from build123d import *

# Parameters (mm, degrees)
SKETCH2_R           = 1.5
CUT_EXTRUDE1_DEPTH  = 10
CUT_EXTRUDE2_DEPTH  = 7
SKETCH4_R           = 2.125
CUT_EXTRUDE4_DEPTH  = 3.5
BOSS_EXTRUDE1_START = 3.7
SKETCH5_R           = 2.1
SKETCH5_R_2         = 1.5
BOSS_EXTRUDE1_DEPTH = 3.7


with BuildPart() as part:
    # Sketch1 → Revolve1 (revolve)
    with BuildSketch(Plane.XY):
        with BuildLine():
            Line((0, 0), (-25, 0))
            ThreePointArc((-25, 0), (-12.85331964, 4.2665982), (0, 5))
            Line((0, 5), (0, 0))
        make_face()
    revolve(axis=Axis((0, 0, 0), (0, 1, 0)))

    # Sketch2 → Cut-Extrude1 (cut)
    with BuildSketch(Plane(origin=(0, 0, 0), x_dir=(-1, 0, 0), z_dir=(0, -1, 0))):
        with Locations(Location((15.4, -10.4, 0), (0, 0, 90))):
            Circle(SKETCH2_R)
        with Locations(Location((-15.4, -10.4, 0), (0, 0, 304.757660669))):
            Circle(SKETCH2_R)
        with Locations(Location((-15.4, 10.4, 0), (0, 0, 90))):
            Circle(SKETCH2_R)
        with Locations(Location((15.4, 10.4, 0), (0, 0, 33.710682562))):
            Circle(SKETCH2_R)
    extrude(amount=-CUT_EXTRUDE1_DEPTH, mode=Mode.SUBTRACT)

    # Sketch3 → Cut-Extrude2 (cut)
    with BuildSketch(Plane(origin=(0, 0, 0), x_dir=(-1, 0, 0), z_dir=(0, -1, 0))):
        with BuildLine():
            Line((11.75, -12.75), (-11.75, -12.75))
            ThreePointArc((-11.75, -12.75), (-12.457106781, -12.457106781), (-12.75, -11.75))
            Line((-12.75, -11.75), (-12.75, 11.75))
            ThreePointArc((-12.75, 11.75), (-12.457106781, 12.457106781), (-11.75, 12.75))
            Line((-11.75, 12.75), (11.75, 12.75))
            ThreePointArc((11.75, 12.75), (12.457106781, 12.457106781), (12.75, 11.75))
            Line((12.75, 11.75), (12.75, -11.75))
            ThreePointArc((12.75, -11.75), (12.457106781, -12.457106781), (11.75, -12.75))
        make_face()
    extrude(amount=-CUT_EXTRUDE2_DEPTH, mode=Mode.SUBTRACT)

    # Sketch4 → Cut-Extrude4 (cut)
    with BuildSketch(Plane(origin=(0, 5, 0), x_dir=(1, 0, 0), z_dir=(0, 1, 0))):
        with Locations(Location((-15.4, 10.4, 0), (0, 0, 270))):
            Circle(SKETCH4_R)
        with Locations(Location((15.4, 10.4, 0), (0, 0, 127.696473345))):
            Circle(SKETCH4_R)
        with Locations(Location((15.4, -10.4, 0), (0, 0, 270))):
            Circle(SKETCH4_R)
        with Locations(Location((-15.4, -10.4, 0), (0, 0, 140.12364515))):
            Circle(SKETCH4_R)
    extrude(amount=-CUT_EXTRUDE4_DEPTH, mode=Mode.SUBTRACT)

    # Sketch5 → Boss-Extrude1 (add)
    # profile 1 of 4: a face of its own
    with BuildSketch(Plane(origin=(0, 0, 0), x_dir=(-1, 0, 0), z_dir=(0, -1, 0)).offset(BOSS_EXTRUDE1_START)):
        with Locations(Location((-15.4, -10.4, 0), (0, 0, 270))):
            Circle(SKETCH5_R)
        with Locations(Location((-15.4, -10.4, 0), (0, 0, 90))):
            Circle(SKETCH5_R_2, mode=Mode.SUBTRACT)
    # profile 2 of 4: a face of its own
    with BuildSketch(Plane(origin=(0, 0, 0), x_dir=(-1, 0, 0), z_dir=(0, -1, 0)).offset(BOSS_EXTRUDE1_START)):
        with Locations(Location((15.4, -10.4, 0), (0, 0, 270))):
            Circle(SKETCH5_R)
        with Locations(Location((15.4, -10.4, 0), (0, 0, 90))):
            Circle(SKETCH5_R_2, mode=Mode.SUBTRACT)
    # profile 3 of 4: a face of its own
    with BuildSketch(Plane(origin=(0, 0, 0), x_dir=(-1, 0, 0), z_dir=(0, -1, 0)).offset(BOSS_EXTRUDE1_START)):
        with Locations(Location((-15.4, 10.4, 0), (0, 0, 270))):
            Circle(SKETCH5_R)
        with Locations(Location((-15.4, 10.4, 0), (0, 0, 90))):
            Circle(SKETCH5_R_2, mode=Mode.SUBTRACT)
    # profile 4 of 4: a face of its own
    with BuildSketch(Plane(origin=(0, 0, 0), x_dir=(-1, 0, 0), z_dir=(0, -1, 0)).offset(BOSS_EXTRUDE1_START)):
        with Locations(Location((15.4, 10.4, 0), (0, 0, 270))):
            Circle(SKETCH5_R)
        with Locations(Location((15.4, 10.4, 0), (0, 0, 90))):
            Circle(SKETCH5_R_2, mode=Mode.SUBTRACT)
    extrude(amount=-BOSS_EXTRUDE1_DEPTH)


solid = part.part
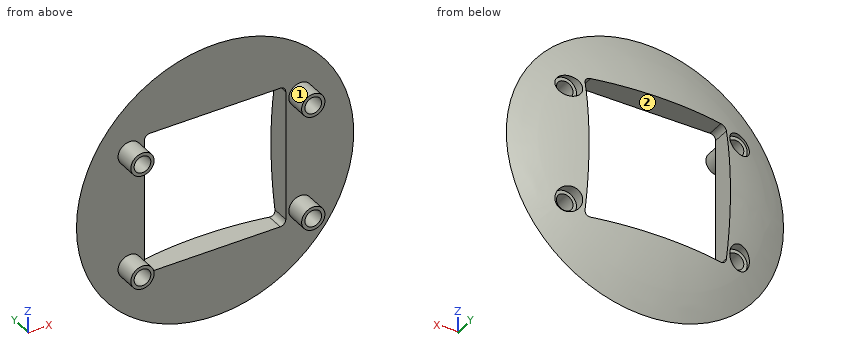
The listing builds one solid part. Answer for the finished solid, in the listing's coordinates (mm). Face numbers are marked on the shaded views. A direction names the side the tool comes from. Give positions to 0.01 mm unless a question says otherwise; leave off trailing zeros. Write each loop counter-clockwise with the first axis right and the second up, starting at its lowest first coordinate (ties: lowest second). Pieces come first, ordered by that corner, then holes. Notation, with made-up numbers: (26, -4.5) -> (34, -4.5) arc R25 ccw to (34, 16.5) -> close; hole circle Ø7 at (-23, 80). An arc over 180 degrees is marked (long way). One line per question, with ' | ' between items. Start each with the question number.
1. Section A-A (y = -2.5) is taken. Determine the outline of the cut face in (x, z), plus the area to 3 significant figures.
2. For the marked faces 1 and 2, determine the directions among +Z, -Z, +X, -X, +Y, -Y from which every point of the face is accessible in a straight line to the end or side of a thin tool.
3. Find the intervals of material crossed by probe 1 along X at (y, z) = (-0.7, 10.4); probe 2 along Z at (x, y) = (-14.5, -0.25); probe 3 along X at (y, z) = (2.3, 10.4) (3 decimals), in increasing order.
4. Given pin 1 Ø4.5 at (x, z) = (-15, 10.5) entering from +Y; pin 2 Ø2 at (y, z) = (2.5, 3) entering from -X; pin 3 Ø2.5 at (x, z) = (15.4, -10.4) entering from +Y; pin 4 Ø15 at (x, z) = (9.5, -0.5) entering from -Y, each flat-ended and moving along its own axis, determine where each tip first touches the part or whether it passes through.
Response values:
1) outline: circle Ø4.2 at (-15.4, -10.4); circle Ø4.2 at (-15.4, 10.4); circle Ø4.2 at (15.4, -10.4); circle Ø4.2 at (15.4, 10.4); hole circle Ø3 at (-15.4, -10.4); hole circle Ø3 at (-15.4, 10.4); hole circle Ø3 at (15.4, -10.4); hole circle Ø3 at (15.4, 10.4) | area: 27.1 mm2
2) face 1: -Y | face 2: +Y, -Y
3) probe 1: -17.5 to -16.9, -13.9 to -13.3, 13.3 to 13.9, 16.9 to 17.5 | probe 2: -12.3 to -11.6, -9.2 to -8.5, 8.5 to 9.2, 11.6 to 12.3 | probe 3: -13.275 to -12.75, 12.75 to 13.275
4) pin 1: y = 3.5 | pin 2: x = -21.61 | pin 3: through | pin 4: y = 0
